Part model, mm, in its own coordinate system. Face numbers are marked on the shaded views. Round coordinates to 2 decimals unless told otherwise and drop trailing zeros. Return JSON: item names as keys, results as strings. Group by question number.
Item 1: Two-plate mould, pull along X, no slides. Class the marked faces 1, 2 and 3: released by +X, released by -X, zero draft, split by the parting line, or undercut.
Item 2: Drop flat-ended pins along their axis: pin 1 (1 mm diameter, centred on y = 10.5, z = 5, fed in from +X); pin 2 (2 mm diameter, centred on x = 2, z = 7, fed in from -Y). Give the stop position or say it passes through.
Item 3: Probe probe 1 along Z at (x, y) = (6, 6.25); probe 2 along X at (y, z) = (10.5, 3.25); probe 3 along X at (y, z) = (9.75, 4.5). List the from-to ranges inside material, lowest first.
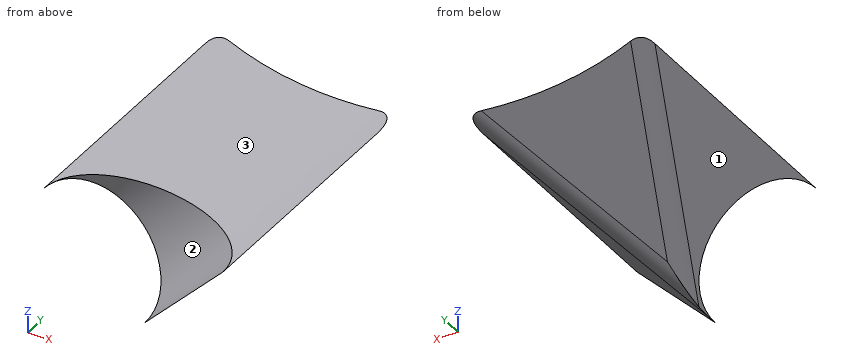
```python
from build123d import *

# Parameters (mm, degrees)
BOSS_EXTRUDE1_DEPTH = 25.4
CUT_EXTRUDE1_REACH  = 30.398
SKETCH2_R           = 6.35
SKETCH4_R           = 83.82
CUT_EXTRUDE3_DEPTH  = 29.398063314
CUT_EXTRUDE4_REACH  = 30.361
FILLET1_R           = 2.54


with BuildPart() as part:
    # Sketch1 → Boss-Extrude1 (new body)
    with BuildSketch(Plane(origin=(0, 0, 0), x_dir=(1, 0, 0), z_dir=(0, 1, 0))):
        Polygon((0, 0), (-8.980256121, -8.980256121), (8.980256121, -8.980256121), align=None)
    extrude(amount=BOSS_EXTRUDE1_DEPTH)

    # Sketch2 → Cut-Extrude1 (cut, up to next)
    with BuildSketch(Plane(origin=(0, 0, 0), x_dir=(-0.7071067811865474, 0, 0.7071067811865477), z_dir=(-0.7071067811865477, 0, -0.7071067811865474)), mode=Mode.PRIVATE) as cut_extrude1_sk1:
        with Locations((6.35, 0)):
            Circle(SKETCH2_R)
    cut_extrude1_tool1 = extrude(cut_extrude1_sk1.sketch, amount=-CUT_EXTRUDE1_REACH, mode=Mode.PRIVATE) & part.part
    add(cut_extrude1_tool1.solids().sort_by_distance((-4.490128, 0, 4.490128))[0], mode=Mode.SUBTRACT)

    # Sketch4 → Cut-Extrude3 (cut, through all)
    with BuildSketch(Plane(origin=(0, 25.4, 0), x_dir=(1, 0, 0), z_dir=(0, 1, 0))):
        with Locations((9.838175311, -90.660480401)):
            Circle(SKETCH4_R)
    extrude(amount=-CUT_EXTRUDE3_DEPTH, mode=Mode.SUBTRACT)

    # Sketch5 → Cut-Extrude4 (cut, up to next)
    with BuildSketch(Plane(origin=(-0.17794868, 0.498418532, -1.352732428), x_dir=(0.9924678045108148, 0.042354141044031964, -0.11495122333366167), z_dir=(0.12250574276124004, -0.3431277622293754, 0.9312656343804265)), mode=Mode.PRIVATE) as cut_extrude4_sk1:
        Polygon((7.123871491, 3.972277825), (-8.869111321, 3.972277825), (-8.869111321, 26.938427805), (7.123871491, 26.216542503), align=None)
    cut_extrude4_tool1 = extrude(cut_extrude4_sk1.sketch, amount=-CUT_EXTRUDE4_REACH, mode=Mode.PRIVATE) & part.part
    add(cut_extrude4_tool1.solids().sort_by_distance((-1.086236, 14.793489, 4.033814))[0], mode=Mode.SUBTRACT)

    # Fillet1
    fillet1_edges = [part.edges().sort_by_distance(p)[0] for p in [
        (3.446132209, 14.816666667, 3.446132209),
        (-4.490128061, 14.816666667, 4.490128061),
    ]]
    fillet(fillet1_edges, radius=FILLET1_R)


solid = part.part
```
Filled in:
{
 "1": {"face 1": "released by -X", "face 2": "undercut", "face 3": "released by +X"},
 "2": {"pin 1": "stops at x = 5.5", "pin 2": "stops at y = 5.08"},
 "3": {"probe 1": "z = 6 to 6.93", "probe 2": "x = -3.23 to 3.25", "probe 3": "x = -4.5 to 4.5"}
}
